```python
from build123d import *

# Parameters (mm, degrees)
SKETCH_1_R          = 4.5
EXTRUDE_1_DEPTH     = 3
SKETCH_2_R          = 2.25
EXTRUDE_2_DEPTH     = 3.5
SKETCH_3_R          = 3.1
EXTRUDE_3_DEPTH     = 4
CHAMFER_1_SIZE      = 0.5
SKETCH_4_W          = 2
SKETCH_4_H          = 10.520514376
CUT_EXTRUDE_1_DEPTH = 2


with BuildPart() as part:
    # Эскиз1 → Бобышка-Вытянуть1 (new body)
    with BuildSketch(Plane.XY):
        Circle(SKETCH_1_R)
    extrude(amount=EXTRUDE_1_DEPTH)

    # Эскиз2 → Бобышка-Вытянуть2 (add)
    with BuildSketch(Plane.XY.offset(3)):
        Circle(SKETCH_2_R)
    extrude(amount=EXTRUDE_2_DEPTH)

    # Эскиз3 → Бобышка-Вытянуть3 (add)
    with BuildSketch(Plane.XY.offset(6.5)):
        Circle(SKETCH_3_R)
    extrude(amount=EXTRUDE_3_DEPTH)

    # Фаска1
    chamfer_1_edges = [part.edges().sort_by_distance(p)[0] for p in [
        (-4.5, 0, 0),
        (-4.5, 0, 3),
        (-3.1, 0, 6.5),
        (-3.1, 0, 10.5),
    ]]
    chamfer(chamfer_1_edges, length=CHAMFER_1_SIZE)

    # Эскиз4 → Вырез-Вытянуть1 (cut)
    with BuildSketch(Plane(origin=(0, 0, 0), x_dir=(-1, 0, 0), z_dir=(0, 0, -1))):
        Rectangle(SKETCH_4_W, SKETCH_4_H)
    extrude(amount=-CUT_EXTRUDE_1_DEPTH, mode=Mode.SUBTRACT)


solid = part.part
```
Part model, mm, in its own coordinate system. A direction names the side the tool comes from. Round coordinates to 2 decimals unless told otherwise and drop trailing zeros. Write each loop counter-clockwise with the first axis right and the second up, starting at its lowest first coordinate (ties: lowest second). Pieces come first, ordered by that corner, then holes.
Item 1: Cut at A-A, the plane x = 0. Give the cut face in (y, z), plus the area to 3 significant figures.
Results:
outline: (-4.5, 2) - (4.5, 2) - (4.5, 2.5) - (4, 3) - (2.25, 3) - (2.25, 6.5) - (2.6, 6.5) - (3.1, 7) - (3.1, 10) - (2.6, 10.5) - (-2.6, 10.5) - (-3.1, 10) - (-3.1, 7) - (-2.6, 6.5) - (-2.25, 6.5) - (-2.25, 3) - (-4, 3) - (-4.5, 2.5) - close
area: 48.8 mm2
Item 2: Probe L1, parallel to Z at x = -0.5, y = 0; L2, parallel to Z at x = 1.25, y = 3.25; L3, parallel to X at y = -4, z = 1.25. List the from-to ranges inside material, lowest first.
Results:
L1: z = 2 to 10.5
L2: z = 0 to 3
L3: x = -2.06 to -1, 1 to 2.06
Item 3: Two-plate mould, pull along X, no slides. Class faces 6 (the flat face through (1, 0, 1)), 7 (the conical face through (4.135, -0.078, 0.135)), 8 (the cylindrical face through (-0.29, 2.23, 4.73)): +X half, -X half, draft (parallel to the pull), parting line (faces both ways), or undercut.
Results:
face 6: undercut
face 7: +X half
face 8: parting line
Item 4: Cut at C-C, the plane y = 0. Give the cut face in (x, z).
Results:
outline: (-4.5, 0.5) - (-4, 0) - (-1, 0) - (-1, 2) - (1, 2) - (1, 0) - (4, 0) - (4.5, 0.5) - (4.5, 2.5) - (4, 3) - (2.25, 3) - (2.25, 6.5) - (2.6, 6.5) - (3.1, 7) - (3.1, 10) - (2.6, 10.5) - (-2.6, 10.5) - (-3.1, 10) - (-3.1, 7) - (-2.6, 6.5) - (-2.25, 6.5) - (-2.25, 3) - (-4, 3) - (-4.5, 2.5) - close
Item 5: Cut at D-D, the plane z = 8.25. Give the cut face in (x, y), plus the area to 3 significant figures.
Results:
outline: circle Ø6.2 at (0, 0)
area: 30.2 mm2
Item 6: Cut at B-B, the plane z = 1.25. Give the cut face in (x, y).
Results:
outline: (-1, -4.39) - (-1, 4.39) arc R4.5 ccw to start; (1, -4.39) arc R4.5 ccw to (1, 4.39) - close
Item 7: Drop flat-ended pins along their axis: pin 1 Ø4 at (y, z) = (1, 6) entering from +X; pin 2 Ø1 at (x, y) = (-2.5, -3.5) entering from +Z; pin 3 Ø1.5 at (x, z) = (2, 5) entering from -Y. Give the stop position or say it passes through.
Results:
pin 1: stops at x = 3.1
pin 2: stops at z = 3
pin 3: stops at y = -1.87
Item 8: Which spindle directions (+Z, -Z, +X, -X, +Y, -Y) get a long thin tool onto all of the face, cutting with end or side? Do faces 1 (the cylindrical face through (4.292, 1.352, 1.486)), 2 (the flat face through (-2, 0, 0)), 3 (the flat face through (-1, 0, 1)), 4 (the flat face through (2, -2, 3)), 5 (the cylindrical face through (1.43, -2.75, 8.48)). Say none if no direction does.
Results:
face 1: +Z, -Z
face 2: -Z, +X, -X, +Y, -Y
face 3: -Z, +Y, -Y
face 4: none
face 5: +Z
